Geometry check sheet. Reference: the model listing, model coordinates, mm. Round coordinates to 2 decimals unless told otherwise and drop trailing zeros. Loops run counter-clockwise (first coordinate to the right, second up) from the corner with the lowest first, then second, coordinate; pieces in that order, holes last.
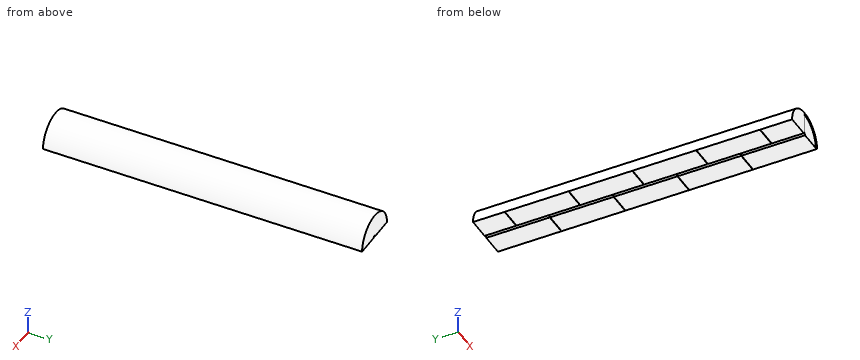
```python
from build123d import *

# Parameters (mm, degrees)
F0_R      = 75
F1_DEPTH  = 1000
F2_R      = 5
F3_DEPTH  = 1000
F5_DEPTH  = 1.2
F8_DEPTH  = 1.2
F26_DEPTH = 1.2
F27_DEPTH = 1.2
F28_DEPTH = 1.2
F29_DEPTH = 1.2
F30_DEPTH = 1.2
F31_DEPTH = 1.2
F32_DEPTH = 1.2
F33_DEPTH = 1.2
F34_W     = 218.629919
F34_H     = 81.904643
F35_DEPTH = 1000


with BuildPart() as f1:
    # F0 (on Front) → F1 (new body)
    with BuildSketch(Plane.XZ):
        Circle(F0_R)
    extrude(amount=-F1_DEPTH)

    # F2 (on Front) → F3 (cut)
    with BuildSketch(Plane.XZ):
        Circle(F2_R)
    extrude(amount=-F3_DEPTH, mode=Mode.SUBTRACT)

    # F4 (on Front) → F5 (cut)
    with BuildSketch(Plane.XZ):
        with BuildLine():
            Line((0, 70), (0, -70))
            ThreePointArc((0, -70), (70, 0), (0, 70))
        make_face()
    extrude(amount=-F5_DEPTH, mode=Mode.SUBTRACT)

    # F7 (on offset) → F8 (cut)
    with BuildSketch(Plane.XZ.offset(-100)):
        with BuildLine():
            Line((0, -70), (0, 70))
            ThreePointArc((0, 70), (-70, 0), (0, -70))
        make_face()
    extrude(amount=-F8_DEPTH, mode=Mode.SUBTRACT)

    # F18 (on offset) → F26 (cut)
    with BuildSketch(Plane.XZ.offset(-200)):
        with BuildLine():
            Line((0, 70), (0, -70))
            ThreePointArc((0, -70), (70, 0), (0, 70))
        make_face()
    extrude(amount=-F26_DEPTH, mode=Mode.SUBTRACT)

    # F19 (on offset) → F27 (cut)
    with BuildSketch(Plane.XZ.offset(-300)):
        with BuildLine():
            Line((0, -70), (0, 70))
            ThreePointArc((0, 70), (-70, 0), (0, -70))
        make_face()
    extrude(amount=-F27_DEPTH, mode=Mode.SUBTRACT)

    # F20 (on offset) → F28 (cut)
    with BuildSketch(Plane.XZ.offset(-400)):
        with BuildLine():
            Line((0, 70), (0, -70))
            ThreePointArc((0, -70), (70, 0), (0, 70))
        make_face()
    extrude(amount=-F28_DEPTH, mode=Mode.SUBTRACT)

    # F21 (on offset) → F29 (cut)
    with BuildSketch(Plane.XZ.offset(-500)):
        with BuildLine():
            Line((0, -70), (0, 70))
            ThreePointArc((0, 70), (-70, 0), (0, -70))
        make_face()
    extrude(amount=-F29_DEPTH, mode=Mode.SUBTRACT)

    # F22 (on offset) → F30 (cut)
    with BuildSketch(Plane.XZ.offset(-600)):
        with BuildLine():
            Line((0, 70), (0, -70))
            ThreePointArc((0, -70), (70, 0), (0, 70))
        make_face()
    extrude(amount=-F30_DEPTH, mode=Mode.SUBTRACT)

    # F23 (on offset) → F31 (cut)
    with BuildSketch(Plane.XZ.offset(-700)):
        with BuildLine():
            Line((0, -70), (0, 70))
            ThreePointArc((0, 70), (-70, 0), (0, -70))
        make_face()
    extrude(amount=-F31_DEPTH, mode=Mode.SUBTRACT)

    # F24 (on offset) → F32 (cut)
    with BuildSketch(Plane.XZ.offset(-800)):
        with BuildLine():
            Line((0, 70), (0, -70))
            ThreePointArc((0, -70), (70, 0), (0, 70))
        make_face()
    extrude(amount=-F32_DEPTH, mode=Mode.SUBTRACT)

    # F25 (on offset) → F33 (cut)
    with BuildSketch(Plane.XZ.offset(-900)):
        with BuildLine():
            Line((0, -70), (0, 70))
            ThreePointArc((0, 70), (-70, 0), (0, -70))
        make_face()
    extrude(amount=-F33_DEPTH, mode=Mode.SUBTRACT)

    # F34 (on Front) → F35 (cut)
    with BuildSketch(Plane.XZ):
        with Locations((-1.260769, -40.952321)):
            Rectangle(F34_W, F34_H)
    extrude(amount=-F35_DEPTH, mode=Mode.SUBTRACT)


solid = f1.part
```
1) Sectioned sample at C-C, the plane z = 32.5. State how many separate pieces and enclosed holes the cut face has, then the cut area to 3 significant figures.
Report:
separate pieces: 1
enclosed holes: 9
area: 134,000 mm2
2) Sectioned sample at B-B, the plane y = 564.5. Record the cut outline in (x, z), then the cut area to 3 significant figures.
Report:
outline: (-75, 0) - (-5, 0) arc R5 cw to (5, 0) - (75, 0) arc R75 ccw to start
area: 8,800 mm2
3) Sectioned sample at A-A, the plane x = -44.5. Record the cut outline in (y, z).
Report:
outline: (0, 0) - (100, 0) - (100, 54.03) - (101.2, 54.03) - (101.2, 0) - (300, 0) - (300, 54.03) - (301.2, 54.03) - (301.2, 0) - (500, 0) - (500, 54.03) - (501.2, 54.03) - (501.2, 0) - (700, 0) - (700, 54.03) - (701.2, 54.03) - (701.2, 0) - (900, 0) - (900, 54.03) - (901.2, 54.03) - (901.2, 0) - (1000, 0) - (1000, 60.37) - (0, 60.37) - close
4) Gauge pin test, flat ends, axial feed: pin 1 (1.3 mm diameter, centred on y = 800.5, z = 23, fed in from +X); pin 2 (6 mm diameter, centred on y = 650, z = 56, fed in from +X); pin 3 (1.5 mm diameter, centred on y = 240.5, z = 9.5, fed in from -X); pin 4 (21 mm diameter, centred on x = -42, z = 40, fed in from -Y). Record the tip position at first contact, or that the pin passes through.
Report:
pin 1: stops at x = 71.59
pin 2: stops at x = 53.07
pin 3: stops at x = -74.49
pin 4: stops at y = 0
5) Scan lines: line 1 along Y through (x, z) = (53.5, 41); line 2 along Y through (x, z) = (-27, 46.5); line 3 along X through (y, z) = (530, 5.5). Record each from-to range of solid material in increasing order.
Report:
line 1: y = 1.2 to 200, 201.2 to 400, 401.2 to 600, 601.2 to 800, 801.2 to 1000
line 2: y = 0 to 100, 101.2 to 300, 301.2 to 500, 501.2 to 700, 701.2 to 900, 901.2 to 1000
line 3: x = -74.8 to 74.8
6) Sectioned sample at D-D, the plane x = 21.5. Record the cut outline in (y, z).
Report:
outline: (0, 66.62) - (1.2, 66.62) - (1.2, 0) - (200, 0) - (200, 66.62) - (201.2, 66.62) - (201.2, 0) - (400, 0) - (400, 66.62) - (401.2, 66.62) - (401.2, 0) - (600, 0) - (600, 66.62) - (601.2, 66.62) - (601.2, 0) - (800, 0) - (800, 66.62) - (801.2, 66.62) - (801.2, 0) - (1000, 0) - (1000, 71.85) - (0, 71.85) - close
